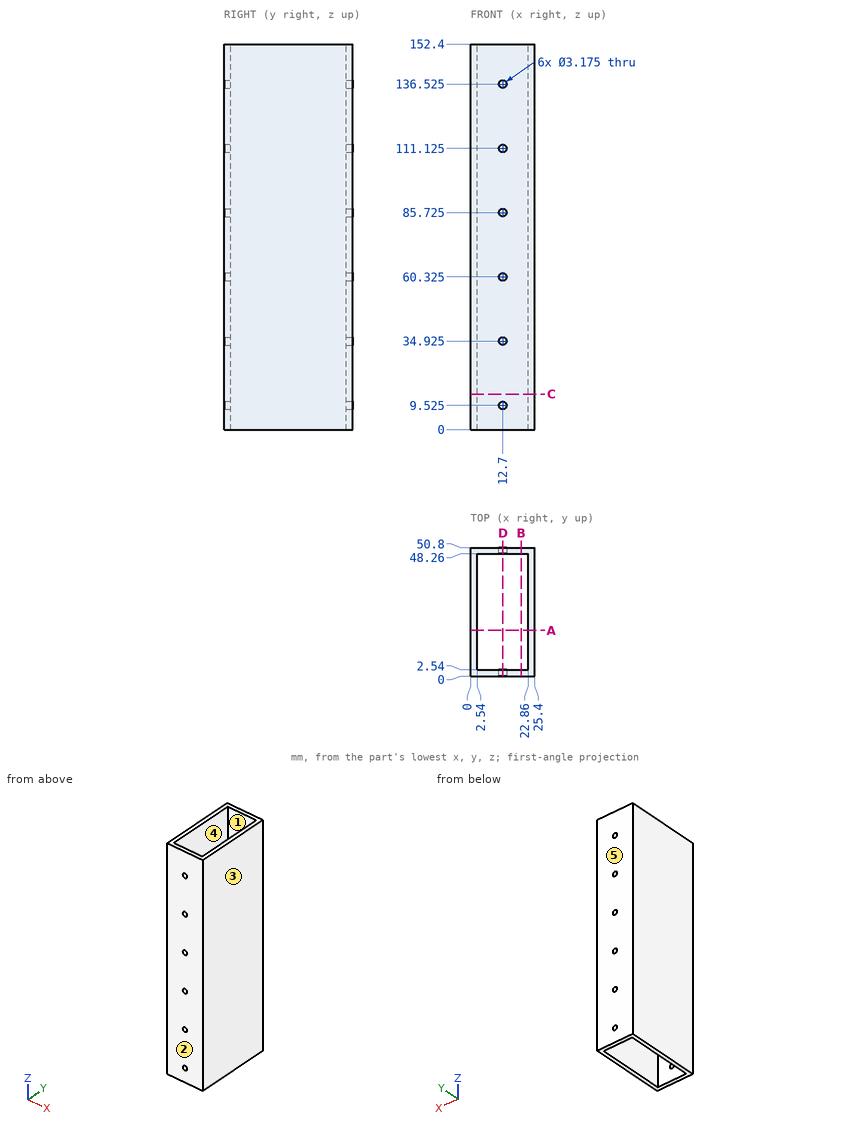
Could you check a few things on this drawing? It's one solid part, dimensions in mm from its lowest x, y, z. A direction names the side the tool comes from. Round coordinates to 2 decimals unless told otherwise and drop trailing zeros. Loops run counter-clockwise (first coordinate to the right, second up) from the corner with the lowest first, then second, coordinate; pieces in that order, holes last. Notation, with made-up numbers: (58.25, 80.5) -> (93.25, 80.5) arc R18 ccw to (93.25, 85.5) -> close; hole circle Ø1 at (-12.75, 30.25). An arc over 180 degrees is marked (long way). One line per item, written item: value. Start each with the question number.
1. If we section it at A-A, the plane y = 18: Write out the boundary of the cut face in (x, z).
2. If I drill on probe 1 along Y at (x, z) = (17.25, 88); probe 2 along X at (y, z) = (48, 106), over which ranges is the centre line in solid material (lowest first)?
3. For the marked faces 1 and 2, which set-ups out of +Z, -Z, +X, -X, +Y, -Y let a thin tool reach every point of the face, with its end or its side?
4. If we section it at B-B, the plane x = 20: Write out the boundary of the cut face in (y, z).
5. If we mould it in two halves opening along Y, with no side actions, what happens to the marked faces 3, 4 and 5? For each: pulls with the +Y half, pulls with the -Y half, needs draft (parallel to the pull), parting line crosses it, or undercut.
6. If we section it at C-C, the plane z = 14: Write out the boundary of the cut face in (x, y).
7. If we section it at D-D, the plane x = 12.7: Give the number of separate pieces and of enclosed holes in the cut face, then the cut area to 3 significant figures.
Calculated:
1. outline: (0, 0) -> (2.54, 0) -> (2.54, 152.4) -> (0, 152.4) -> close; (22.86, 0) -> (25.4, 0) -> (25.4, 152.4) -> (22.86, 152.4) -> close
2. probe 1: y = 0 to 2.54, 48.26 to 50.8
2. probe 2: x = 0 to 2.54, 22.86 to 25.4
3. face 1: +Z, -Z
3. face 2: +Z, -Z, +X, -X, -Y
4. outline: (0, 0) -> (2.54, 0) -> (2.54, 152.4) -> (0, 152.4) -> close; (48.26, 0) -> (50.8, 0) -> (50.8, 152.4) -> (48.26, 152.4) -> close
5. face 3: needs draft
5. face 4: undercut
5. face 5: pulls with the +Y half
6. outline: (0, 0) -> (25.4, 0) -> (25.4, 50.8) -> (0, 50.8) -> close; hole (2.54, 2.54) -> (22.86, 2.54) -> (22.86, 48.26) -> (2.54, 48.26) -> close
7. separate pieces: 14
7. enclosed holes: 0
7. area: 677 mm²
